The listing builds one solid part. Answer for the finished solid, in the listing's coordinates (mm). A direction names the side the tool comes from. Coordinates: 2 decimals unless noted, no trailing zeros. Write each loop counter-clockwise with the first axis right and the second up, starting at its lowest first coordinate (ties: lowest second). Pieces come first, ordered by that corner, then holes.
(1) Given P1, Ø3, axis at x = 1.5, z = 3.5, coming from the -Y side; P2, Ø2, axis at x = 0.5, z = 6, coming from the +Y side; P3, Ø1.5, axis at y = -2.5, z = 8.5, coming from the +X side, each flat-ended and moving along its own axis, determine where each tip first touches the part or whether it passes through.
(2) Which of the six approach directions +Z, -Z, +X, -X, +Y, -Y give full straight-line access (tool end or side, diameter ignored) to faces 1 (the flat face through (2.285, 1.293, -3.046)), 2 (the flat face through (1.1, -2.4, 0)), 3 (the flat face through (0, 0, 12.7))?
(3) The part is cut by section B-B on z = 1.5. Determine the outline of the cut face in (x, y), plus the area to 3 significant figures.
(4) Straight lines are drawn through the part: line 1 (Z direction, x = -1, y = -1.25); line 2 (Z direction, x = -2.5, y = 2) (3 decimals); line 3 (Y direction, x = -1.25, z = 10.25). For each, find the intervals that lie inside material, in ascending order.
(5) For a pull along X with two mould halves and no side action, classify faces 4 (the flat face through (0, -3, -3.175)), 5 (the flat face through (2.175, 1.233, -2.107)), 6 (the cylindrical face through (-0.31, -2.33, 6.26)) as +X half, -X half, draft (parallel to the pull), parting line (faces both ways), or undercut.
Autodesk Inventor part; units mm, degrees
ref_plane "YZ Plane" through (0, 0, 0) normal (1, 0, 0) x (0, 1, 0)
ref_plane "XZ Plane" through (0, 0, 0) normal (0, 1, 0) x (-1, 0, 0)
ref_plane "XY Plane" through (0, 0, 0) normal (0, 0, 1) x (1, 0, 0)
sketch "Sketch1" plane through (0, 0, 0) normal (0, 0, 1) x (1, 0, 0)
  circle A0 centre (0, 0) radius 5.763
  circle A1 centre (0, 0) radius 2.3495
  line L0 (2.8868, 0) -> (1.4434, -2.5)
  line L1 (1.4434, -2.5) -> (-1.4434, -2.5)
  line L2 (-1.4434, -2.5) -> (-2.8868, 0)
  line L3 (-2.8868, 0) -> (-1.4434, 2.5)
  line L4 (-1.4434, 2.5) -> (1.4434, 2.5)
  line L5 (1.4434, 2.5) -> (2.8868, 0)
  dimension "d0" = 11.526
  dimension "d2" = 4.699
  dimension "d5" = 5
extrude "Extrusion1" add sketch "Sketch1" along normal blind 12.7 contours A1
extrude "Extrusion2" add sketch "Sketch1" against normal blind 3.175 contours A0 | A1 | L0 L1 L2 L3 L4 L5
fillet "Fillet1" radius 2.54 1 edges at (-5.763, 0, -3.175)
sketch "Sketch2" plane through (0, 0, -3.175) normal (0, 0, -1) x (-1, 0, 0)
  circle A0 centre (0, 0) radius 2.3495
  circle A1 centre (0, 0) radius 3.223
  line L0 (2.8868, 0) -> (1.4434, -2.5)
  line L1 (1.4434, -2.5) -> (-1.4434, -2.5)
  line L2 (-1.4434, -2.5) -> (-2.8868, 0)
  line L3 (-2.8868, 0) -> (-1.4434, 2.5)
  line L4 (-1.4434, 2.5) -> (1.4434, 2.5)
  line L5 (1.4434, 2.5) -> (2.8868, 0)
  dimension "d9" = 5
extrude "Extrusion3" cut sketch "Sketch2" against normal blind 1.905 contours A0 | L0 L1 L2 L3 L4 L5
thread "Thread1"
chamfer "Chamfer1" distance 0.254 angle 45 7 edges at (2.1651, 1.25, -3.175) (0, 2.5, -3.175) (-2.1651, 1.25, -3.175) (2.1651, -1.25, -3.175) (0, -2.5, -3.175) (-2.1651, -1.25, -3.175) (-5.763, 0, 0)
properties part number "10-32 Bolt" material "Steel"
Model answer:
1. P1: stops at y = -2.35
1. P2: stops at y = 2.35
1. P3: stops at x = 1.57
2. face 1: -Z
2. face 2: +Z
2. face 3: +Z, +X, -X, +Y, -Y
3. outline: circle Ø4.7 at (0, 0)
3. area: 17.3 mm2
4. line 1: z = -1.27 to 12.7
4. line 2: z = -3.175 to 0
4. line 3: y = -1.99 to 1.99
5. face 4: draft
5. face 5: undercut
5. face 6: parting line
